Work out the finished part from the listing and answer in its coordinate system (mm). Face numbers are marked on the shaded views. A direction names the side the tool comes from. Round coordinates to 2 decimals unless told otherwise and drop trailing zeros. Loops run counter-clockwise (first coordinate to the right, second up) from the corner with the lowest first, then second, coordinate; pieces in that order, holes last. Notation, with made-up numbers: (-21.5, 14) - (-1.5, 14) arc R12 cw to (-1.5, 25) - close; hole circle Ø7 at (-1, 56.5). An arc over 180 degrees is marked (long way). Return JSON: item names as keys, results as strings.
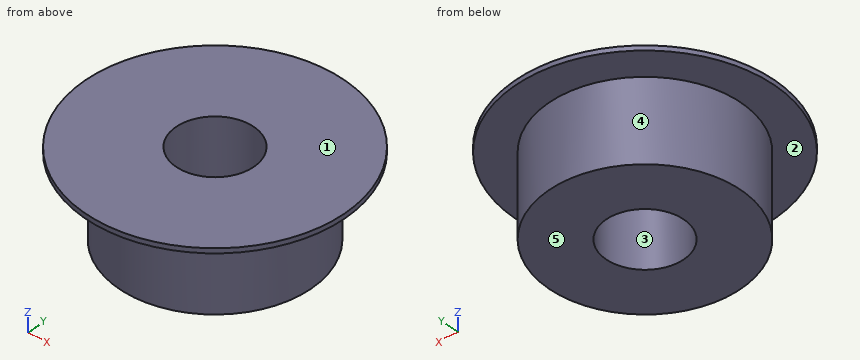
from build123d import *

# Parameters (mm, degrees)
F0_R     = 10
F1_DEPTH = 8.5
F2_R     = 10
F2_R_2   = 13.5
F3_DEPTH = 0.5
F4_R     = 4.05
F5_DEPTH = 9.001


with BuildPart() as f1:
    # F0 (on Top) → F1 (new body)
    with BuildSketch(Plane.XY):
        Circle(F0_R)
    extrude(amount=F1_DEPTH)

    # F2 (on face) → F3 (join)
    with BuildSketch(Plane.XY.offset(8.5)):
        Circle(F2_R)
        Circle(F2_R_2)
        Circle(F2_R, mode=Mode.SUBTRACT)
        Circle(F2_R_2)
    extrude(amount=F3_DEPTH)

    # F4 (on face) → F5 (cut, through all)
    with BuildSketch(Plane.XY.offset(9)):
        Circle(F4_R)
    extrude(amount=-F5_DEPTH, mode=Mode.SUBTRACT)


solid = f1.part
1) Find the intervals of material crossed by L1, parallel to Y at x = 0, z = 7; L2, parallel to Z at x = -9.25, y = -5.25; L3, parallel to X at y = -3.5, z = 4.25, in increasing order.
Verdict:
{"L1": "y = -10 to -4.05, 4.05 to 10", "L2": "z = 8.5 to 9", "L3": "x = -9.37 to -2.04, 2.04 to 9.37"}
2) A tool of negligible diameter and unlimited length cuts with its end or side. For the marked faces 1 and 2, from which of +Z, -Z, +X, -X, +Y, -Y can it reach the whole face along a straight path? Write none if from no direction.
Verdict:
{"face 1": "+Z, +X, -X, +Y, -Y", "face 2": "-Z"}
3) Flat-ended cylindrical pins translate along their axes: pin 1 (2 mm diameter, centred on x = 1.5, z = 4, fed in from -Y); pin 2 (3 mm diameter, centred on y = -1, z = 5, fed in from -X); pin 3 (1 mm diameter, centred on x = 9.5, z = 6.5, fed in from -Y). Find the tip coordinate at first contact, or state that the pin passes through.
Verdict:
{"pin 1": "stops at y = -9.99", "pin 2": "stops at x = -10", "pin 3": "stops at y = -4.36"}
4) Section D-D (x = 7.5) is taken. Give the vertices of the cut face in (y, z).
Verdict:
{"outline": "(-11.22, 8.5) - (-6.61, 8.5) - (-6.61, 0) - (6.61, 0) - (6.61, 8.5) - (11.22, 8.5) - (11.22, 9) - (-11.22, 9) - close"}
5) Determine the mould class of the marked faces 3, 4 and 5 for opening direction X: pulls with the +X half, pulls with the -X half, needs draft (parallel to the pull), parting line crosses it, or undercut.
Verdict:
{"face 3": "undercut", "face 4": "parting line crosses it", "face 5": "needs draft"}
6) Section C-C (z = 6.25) is taken. Give the vertices of the cut face in (x, y).
Verdict:
{"outline": "circle Ø20 at (0, 0); hole circle Ø8.1 at (0, 0)"}
7) Section A-A (y = 0) is taken. Give the vertices of the cut face in (x, z), and give its area (3 significant figures).
Verdict:
{"outline": "(-13.5, 8.5) - (-10, 8.5) - (-10, 0) - (-4.05, 0) - (-4.05, 9) - (-13.5, 9) - close; (4.05, 0) - (10, 0) - (10, 8.5) - (13.5, 8.5) - (13.5, 9) - (4.05, 9) - close", "area": "111 mm2"}
